Here's how the part is built. I have some questions about the finished solid (model axes, mm). A direction names the side the tool comes from. Give positions to 0.01 mm unless a question says otherwise; leave off trailing zeros. Order: outer loops, then holes, each group sorted by start corner. A loop starts at its lowest first (then second) coordinate and runs counter-clockwise, first axis right, second up. Notation, with made-up numbers: (53.5, -31.75) -> (78.5, -31.75) arc R18 ccw to (78.5, -21.75) -> close; hole circle Ø3 at (-18, 44). An arc over 180 degrees is marked (long way). Write each question's results on one line, items separated by ' | '. Start each with the question number.
Q1. Thinking about a two-plate mould opening in Y: for faces 1 (the face through (9, -9, -0.755)), 2 (the face through (-9, -13, -17.5)), which applies, pulls with the +Y half, pulls with the -Y half, needs draft (parallel to the pull), parting line crosses it, or undercut?
Q2. Imagine slicing it at B-B, the plane x = 0. State how many separate pieces and enclosed holes the cut face has, then the cut area to 3 significant figures.
Q3. For faces 3 (the face through (13.18, -3.15, -3.3)), 4 (the face through (-17.07, 6.714, -11.837)), 5 (the face through (-11, 17, 4.245)), which set-ups out of +Z, -Z, +X, -X, +Y, -Y let a thin tool reach every point of the face, with its end or its side?
Q4. I need wall thicknesses on line 1 along X through (y, z) = (-16, 3.25); line 2 along Y through (x, z) = (0, -3) (3 decimals); line 3 along Z through (x, y) = (1, 15). Which ranges of each line are inside material? Lowest first, please. Write a range as [from, to].
Q5. Imagine slicing it at A-A, the plane z = -14.75. Please give me the cut outline in (x, y) (3 decimals).
Q6. Imagine slicing it at C-C, the plane z = -8. Please give me the cut outline in (x, y) (3 decimals).
Q7. I'm going to push flat-ended pins straight in: pin 1 (8.5 mm diameter, centred on x = -9.33, y = 12.84, fed in from +Z); pin 2 (1 mm diameter, centred on y = -12.5, z = -2, fed in from -X); pin 3 (2 mm diameter, centred on y = -9, z = -7, fed in from +X). Where does each tip first touch, or does it pass through?
```python
from build123d import *
from build123d.topology import SkipClean

# Parameters (mm, degrees)
SKETCH_10_R             = 2.675
EXTRUDE_5_DEPTH         = 17.5
CHAMFER1_SIZE           = 1
CHAMFER1_SIZE2          = 1.017920191
SKETCH_4_R              = 12.5
CUT_EXTRUDE_1_DEPTH     = 44.106650761
HOLE_WIZARD_M5_1_D      = 5.2
CIRPATTERN1_START       = -7.186794992
CIRPATTERN1_5_OUTLINE_R = 2.6
CIRPATTERN1_5_DEPTH     = 11.431671907
SKETCH_14_W             = 5
SKETCH_14_H             = 20
BOSS_EXTRUDE1_START     = 0.4
SKETCH1_R               = 28.255495976
SKETCH1_R_2             = 20
BOSS_EXTRUDE1_DEPTH     = 0.4
SKETCH4_R               = 25
CUT_EXTRUDE3_DEPTH      = 0.4
FILLET1_R               = 2


# Read off the part's stored shape, not the designer's step: 구배1, CirPattern1
with BuildPart() as part:
    # 스케치7 → 회전2 (revolve)
    with BuildSketch(Plane.ZY, mode=Mode.PRIVATE) as revolve_2_sk:
        with BuildLine():
            ThreePointArc((2.354808499, 29.346727485), (0.845544662, 25.810608837), (0, 22.06))
            Line((0, 22.06), (4.244876915, 22.06))
            Line((4.244876915, 22.06), (4.244876915, 28.255495976))
            Line((4.244876915, 28.255495976), (2.354808499, 29.346727485))
        make_face()
        with BuildLine():
            Line((-7.405123085, 11), (-7.405123085, 0))
            Line((-7.405123085, 0), (4.244876915, 0))
            Line((4.244876915, 0), (4.244876915, 22.06))
            Line((4.244876915, 22.06), (0, 22.06))
            ThreePointArc((0, 22.06), (-5.382911125, 17.655062883), (-7.405123085, 11))
        make_face()
    revolve(revolve_2_sk.sketch.rotate(Axis((0, 0, -7.405123085), (0, 0, 1)), 90), axis=Axis((0, 0, -7.405123085), (0, 0, 1)))

    # 스케치10 → 보스-돌출5 (add)
    with BuildSketch(Plane.XY):
        with Locations((0, 15.875)):
            Circle(SKETCH_10_R)
    extrude(amount=-EXTRUDE_5_DEPTH)

    # 구배1 outline → 구배1 (revolve)
    with BuildSketch(Plane.XZ.offset(-15.875)):
        Polygon((2.675, -17.5), (2.901355148, -4.532122261), (2.675, -4.532122261), align=None)
    revolve(axis=Axis((0, 15.875, 0), (0, 0, 1)))

    # Chamfer1
    chamfer1_edges = [part.edges().sort_by_distance(p)[0] for p in [
        (-2.675, 15.875, -17.5),
    ]]
    chamfer1_side = [part.faces().sort_by_distance(p)[0] for p in [
        (0, 15.875, -17.5),
    ]]
    chamfer(chamfer1_edges, length=CHAMFER1_SIZE, length2=CHAMFER1_SIZE2, reference=chamfer1_side[0])

    # 스케치4 → 컷-돌출1 (cut, through all)
    with BuildSketch(Plane(origin=(0, 0, -7.405123085), x_dir=(-1, 0, 0), z_dir=(0, 0, -1))):
        with Locations(Location((0, 0, 0), (0, 0, 90))):
            Circle(SKETCH_4_R)
    extrude(amount=-CUT_EXTRUDE_1_DEPTH, mode=Mode.SUBTRACT)

    # M5 나선 코일용 탭 드릴1 (through all)
    with Locations(Plane.XY.offset(4.244876915)):
        with Locations((0, -15.875)):
            Hole(HOLE_WIZARD_M5_1_D / 2)

    # CirPattern1 outline → CirPattern1 (revolve)
    with BuildSketch(Plane(origin=(15.098022196, 4.905644786, 0), x_dir=(1, 0, 0), z_dir=(0, -1, 0))):
        Polygon((0, -4.72112791), (0, -17.5), (1.675, -17.5), (2.675, -16.5), (2.675, -4.72112791), align=None)
    revolve(axis=Axis((15.098022196, 4.905644786, 0), (0, 0, 1)))

    # CirPattern1 2 outline → CirPattern1 2 (revolve)
    with BuildSketch(Plane(origin=(9.33109088, -12.843144786, 0), x_dir=(1, 0, 0), z_dir=(0, -1, 0))):
        Polygon((0, -4.721045305), (0, -17.5), (1.675, -17.5), (2.675, -16.5), (2.675, -4.721045305), align=None)
    revolve(axis=Axis((9.33109088, -12.843144786, 0), (0, 0, 1)))

    # CirPattern1 3 outline → CirPattern1 3 (revolve)
    with BuildSketch(Plane(origin=(-9.33109088, -12.843144786, 0), x_dir=(1, 0, 0), z_dir=(0, -1, 0))):
        Polygon((0, -4.72095341), (0, -17.5), (1.675, -17.5), (2.675, -16.5), (2.675, -4.72095341), align=None)
    revolve(axis=Axis((-9.33109088, -12.843144786, 0), (0, 0, 1)))

    # CirPattern1 4 outline → CirPattern1 4 (revolve)
    with BuildSketch(Plane(origin=(-15.098022196, 4.905644786, 0), x_dir=(1, 0, 0), z_dir=(0, -1, 0))):
        Polygon((0, -4.721296369), (0, -17.5), (1.675, -17.5), (2.675, -16.5), (2.675, -4.721296369), align=None)
    revolve(axis=Axis((-15.098022196, 4.905644786, 0), (0, 0, 1)))

    # CirPattern1 5 outline → CirPattern1 5 (cut)
    with BuildSketch(Plane.XY.offset(CIRPATTERN1_START)):
        with Locations((-15.098022196, -4.905644786)):
            Circle(CIRPATTERN1_5_OUTLINE_R)
        with Locations((-9.33109088, 12.843144786)):
            Circle(CIRPATTERN1_5_OUTLINE_R)
        with Locations((9.33109088, 12.843144786)):
            Circle(CIRPATTERN1_5_OUTLINE_R)
        with Locations((15.098022196, -4.905644786)):
            Circle(CIRPATTERN1_5_OUTLINE_R)
    extrude(amount=CIRPATTERN1_5_DEPTH, mode=Mode.SUBTRACT)

    # 스케치14 → 컷-회전1 (revolve, cut)
    with BuildSketch(Plane(origin=(0, 0, 0), x_dir=(0, 0, -1), z_dir=(1, 0, 0))):
        with Locations((-1.744876915, 10)):
            Rectangle(SKETCH_14_W, SKETCH_14_H)
    revolve(axis=Axis((0, 0, 4.244876915), (0, 0, -1)), mode=Mode.SUBTRACT)

    # Sketch1 → Boss-Extrude1 (add)
    with SkipClean():  # the faces are left unmerged after this step: merging them gives an invalid solid
        with BuildSketch(Plane.XY.offset(4.244876915).offset(BOSS_EXTRUDE1_START)):
            Circle(SKETCH1_R)
            Circle(SKETCH1_R_2, mode=Mode.SUBTRACT)
        extrude(amount=-BOSS_EXTRUDE1_DEPTH)

    # Sketch4 → Cut-Extrude3 (cut)
    with BuildSketch(Plane.XY.offset(4.644876915)):
        Circle(SKETCH4_R)
    extrude(amount=-CUT_EXTRUDE3_DEPTH, mode=Mode.SUBTRACT)

    # Fillet1
    # the kernel refuses this fillet: 2 mm, written as the material it adds along each edge
    with BuildSketch(Plane(origin=(0, 0, 4.244876915), x_dir=(-1, 0, 0), z_dir=(0, 1, 0))) as fillet1_piece_1:
        with BuildLine():
            CenterArc((30.250231597, 0.545016556), FILLET1_R, 184.158067237, 25.841932763)
            Line((28.518180789, -0.454983444), (28.483539773, -0.474983444))
            Line((28.483539773, -0.474983444), (28.22085496, -0.02))
            Line((28.22085496, -0.02), (28.215495976, 0))
            ThreePointArc((28.215495976, 0), (28.215495976, 0.2), (28.215601263, 0.397099669))
            Line((28.215601263, 0.397099669), (28.255495976, 0.4))
        make_face()
    revolve(axis=Axis((0, 0, 4.244876915), (0, 0, 1)), revolution_arc=180)
    with BuildSketch(Plane(origin=(0, 0, 4.244876915), x_dir=(1, 0, 0), z_dir=(0, -1, 0))) as fillet1_piece_2:
        with BuildLine():
            CenterArc((30.250231597, 0.545016556), FILLET1_R, 184.158067237, 25.841932763)
            Line((28.518180789, -0.454983444), (28.483539773, -0.474983444))
            Line((28.483539773, -0.474983444), (28.22085496, -0.02))
            Line((28.22085496, -0.02), (28.215495976, 0))
            ThreePointArc((28.215495976, 0), (28.215495976, 0.2), (28.215601263, 0.397099669))
            Line((28.215601263, 0.397099669), (28.255495976, 0.4))
        make_face()
    revolve(axis=Axis((0, 0, 4.244876915), (0, 0, 1)), revolution_arc=180)


solid = part.part
```
Geometry check:
1) face 1: undercut | face 2: needs draft
2) separate pieces: 3 | enclosed holes: 0 | area: 184 mm²
3) face 3: +Z, -Z | face 4: -Z | face 5: +Z
4) line 1: [-23.98, -12], [12, 23.98] | line 2: [-20.273, -18.475], [-13.275, -12.5], [12.5, 20.273] | line 3: [-17.5, -0.76]
5) outline: circle Ø5.35 at (-15.098, 4.906); circle Ø5.35 at (-9.331, -12.843); circle Ø5.446 at (0, 15.875); circle Ø5.35 at (9.331, -12.843); circle Ø5.35 at (15.098, 4.906)
6) outline: circle Ø5.35 at (-15.098, 4.906); circle Ø5.35 at (-9.331, -12.843); circle Ø5.682 at (0, 15.875); circle Ø5.35 at (9.331, -12.843); circle Ø5.35 at (15.098, 4.906)
7) pin 1: z = 4.24 | pin 2: x = -17.41 | pin 3: x = 14.07
